Geometry: final body of the model. Coordinates: model frame, mm. A direction names the side the tool comes from. Give positions to 0.01 mm unless a question says otherwise; leave off trailing zeros. Order: outer loops, then holes, each group sorted by start corner. A loop starts at its lowest first (then second) coordinate and runs counter-clockwise, first axis right, second up. Notation, with made-up numbers: M 77,83 L 136,83 A35 cw 136,119 Z; hole C 58.5,31 d3. An arc over 180 degrees is marked long. One line per item, written item: value. Start each with the question number.
```python
from build123d import *

# Parameters (mm, degrees)
ESQUISSE1_R             = 38.1
BOSS_EXTRU_1_DEPTH      = 11
ESQUISSE2_R             = 19.05
BOSS_EXTRU_2_DEPTH      = 19
ESQUISSE3_R             = 3.175
ENL_V_MAT_EXTRU_1_DEPTH = 31


with BuildPart() as part:
    # Esquisse1 → Boss.-Extru.1 (new body)
    with BuildSketch(Plane(origin=(0, 0, 0), x_dir=(1, 0, 0), z_dir=(0, 1, 0))):
        Circle(ESQUISSE1_R)
    extrude(amount=BOSS_EXTRU_1_DEPTH)

    # Esquisse2 → Boss.-Extru.2 (add)
    with BuildSketch(Plane(origin=(0, 11, 0), x_dir=(1, 0, 0), z_dir=(0, 1, 0))):
        Circle(ESQUISSE2_R)
    extrude(amount=BOSS_EXTRU_2_DEPTH)

    # Esquisse3 → Enlèv. mat.-Extru.1 (cut, through all)
    with BuildSketch(Plane(origin=(0, 30, 0), x_dir=(1, 0, 0), z_dir=(0, 1, 0))):
        Circle(ESQUISSE3_R)
    extrude(amount=-ENL_V_MAT_EXTRU_1_DEPTH, mode=Mode.SUBTRACT)


solid = part.part
```
Q1. Section query A-A on z = 0. Return loops of the section in (x, y) (3 decimals), and give its area (3 significant figures).
Q2. Mould query, pull axis X, two halves, no side actions, for faces 3 (the face through (-0.69, 15.21, 3.1)), 4 (the face through (-30.235, 5.423, 23.183)), 5 (the face through (7.9, 11, -17.5)). Classes: +X half, -X half, draft (parallel to the pull), parting line (faces both ways), or undercut.
Q3. Set-up query: faces 1 (the face through (-15.12, 20.37, 11.59)), 2 (the face through (8, 0, -1)). Return all of +Z, -Z, +X, -X, +Y, -Y with unobstructed straight access to the full face (end or side cutting, diameter ignored); none if empty.
Q4. Ray query, line 1 along X through (y, z) = (8, 0) (3 decimals); line 2 along Z through (x, y) = (0, 17) (3 decimals). Return the intervals inside material, ascending. Write a range as [from, to].
Q5. Section query B-B on x = 0. Return loops of the section in (y, z) (3 decimals), and give its area (3 significant figures).
Q6. Section query C-C on y = 19.75. Return loops of the section in (x, z) (3 decimals), and give its area (3 significant figures).
Q7. Section query D-D on x = 10. Return loops of the section in (y, z), and give its area (3 significant figures).
Q8. Contact query for flat-ended pins moving along their axis: pin 1 (5 mm diameter, centred on y = 26, z = -6, fed in from -X); pin 2 (2 mm diameter, centred on y = 5.5, z = 3.5, fed in from -X); pin 3 (10 mm diameter, centred on x = 29, y = 16.5, fed in from -Z); pin 4 (10 mm diameter, centred on y = 18, z = -14, fed in from +X). Output: stop coordinate, or through.
Results below:
1. outline: M -38.1,0 L -3.175,0 L -3.175,30 L -19.05,30 L -19.05,11 L -38.1,11 Z; M 3.175,0 L 38.1,0 L 38.1,11 L 19.05,11 L 19.05,30 L 3.175,30 Z
1. area: 1,370 mm2
2. face 3: undercut
2. face 4: parting line
2. face 5: draft
3. face 1: +Y
3. face 2: +Z, -Z, +X, -X, -Y
4. line 1: [-38.1, -3.175], [3.175, 38.1]
4. line 2: [-19.05, -3.175], [3.175, 19.05]
5. outline: M 0,-38.1 L 11,-38.1 L 11,-19.05 L 30,-19.05 L 30,-3.175 L 0,-3.175 Z; M 0,3.175 L 30,3.175 L 30,19.05 L 11,19.05 L 11,38.1 L 0,38.1 Z
5. area: 1,370 mm2
6. outline: C 0,0 d38.1; hole C 0,0 d6.35
6. area: 1,110 mm2
7. outline: M 0,-36.76 L 11,-36.76 L 11,-16.21 L 30,-16.21 L 30,16.21 L 11,16.21 L 11,36.76 L 0,36.76 Z
7. area: 1,420 mm2
8. pin 1: x = -18.73
8. pin 2: x = -38.02
8. pin 3: through
8. pin 4: x = 16.79
